```python
from build123d import *

# Parameters (mm, degrees)
BOSS_EXTRUDE1_DEPTH                           = 63.5
F_18_0_18_DIAMETER_HOLE1_D                    = 18
CBORE_FOR_4_SOCKET_HEAD_CAP_SCREW1_AT_2_COUNT = 2
CBORE_FOR_4_SOCKET_HEAD_CAP_SCREW1_AT_2_PITCH = 38.572873922
M5_CLEARANCE_HOLE1_D                          = 5.5
CBORE_FOR_5_16_HEX_MACHINE_SCREW1_D           = 8.4328
CBORE_FOR_5_16_HEX_MACHINE_SCREW1_CBORE_D     = 20.6375
CBORE_FOR_5_16_HEX_MACHINE_SCREW1_CBORE_DEPTH = 5.842
F_10_CLEARANCE_HOLE1_D                        = 5.1054
CUT_EXTRUDE1_DEPTH                            = 27.19375
CUT_EXTRUDE1_DEPTH_BACK                       = 27.19375


with BuildPart() as part:
    # Sketch1 → Boss-Extrude1 (new body)
    with BuildSketch(Plane.XY):
        Polygon((-26.19375, 0), (26.19375, 0), (26.19375, 9.525), (26.19375, 85.725), (19.05, 85.725), (19.05, 9.525), (-19.05, 9.525), (-19.05, 85.725), (-26.19375, 85.725), (-26.19375, 9.525), align=None)
    extrude(amount=BOSS_EXTRUDE1_DEPTH)

    # 18.0 _18_ Diameter Hole1 (through all)
    with Locations(Plane(origin=(26.19375, 0, 0), x_dir=(0, 0, -1), z_dir=(1, 0, 0))):
        with Locations((-28.575, 42.8625)):
            Hole(F_18_0_18_DIAMETER_HOLE1_D / 2)

    # Sketch13 → CBORE for _4 Socket Head Cap Screw1 (revolve, cut)
    with BuildSketch(Plane(origin=(-26.19375, 61.9125, 12.7), x_dir=(0, 0, 1), z_dir=(0, 1, 0))):
        Polygon((0, 0), (0, 42.382574487), (1.63195, 41.402), (1.63195, 2.8448), (2.77876, 2.8448), (2.77876, 0), align=None)
    cbore_for_4_socket_head_cap_screw1 = revolve(axis=Axis((-32.54375, 61.9125, 12.7), (1, 0, 0)), mode=Mode.SUBTRACT)

    # CBORE for _4 Socket Head Cap Screw1 at 2: CBORE for _4 Socket Head Cap Screw1 ×2
    with Locations(*[Vector(0, -0.195090322, 0.98078528) * (i * CBORE_FOR_4_SOCKET_HEAD_CAP_SCREW1_AT_2_PITCH) for i in range(1, CBORE_FOR_4_SOCKET_HEAD_CAP_SCREW1_AT_2_COUNT)]):
        add(cbore_for_4_socket_head_cap_screw1, mode=Mode.SUBTRACT)

    # Mirror1: CBORE for _4 Socket Head Cap Screw1 across Right Plane
    add(cbore_for_4_socket_head_cap_screw1.mirror(Plane(origin=(0, 0, 0), x_dir=(0, 0, -1), z_dir=(1, 0, 0))), mode=Mode.SUBTRACT)

    # Mirror1 copy 1 sketch → Mirror1 copy 1 (revolve, cut)
    with BuildSketch(Plane(origin=(26.19375, 54.387305606, 50.531706965), x_dir=(0, 0, 1), z_dir=(0, 1, 0))):
        Polygon((0, 0), (0, -42.382574487), (1.63195, -41.402), (1.63195, -2.8448), (2.77876, -2.8448), (2.77876, 0), align=None)
    revolve(axis=Axis((32.54375, 54.387305606, 50.531706965), (1, 0, 0)), mode=Mode.SUBTRACT)

    # M5 Clearance Hole1 (through all)
    with Locations(Plane.ZY.offset(26.19375)):
        with Locations((28.575, 67.862500038), (28.575, 17.862499962)):
            m5_clearance_hole1 = Hole(M5_CLEARANCE_HOLE1_D / 2)

    # Mirror2: M5 Clearance Hole1 across plane
    add(m5_clearance_hole1.mirror(Plane(origin=(0, 0, 0), x_dir=(0, 0, 1), z_dir=(1, 0, 0))), mode=Mode.SUBTRACT)

    # CBORE for 5_16 Hex Machine Screw1 (through all)
    with Locations(Plane(origin=(0, 9.525, 0), x_dir=(1, 0, 0), z_dir=(0, 1, 0))):
        with Locations((0, -47.625), (0, -15.875)):
            CounterBoreHole(CBORE_FOR_5_16_HEX_MACHINE_SCREW1_D / 2, CBORE_FOR_5_16_HEX_MACHINE_SCREW1_CBORE_D / 2, CBORE_FOR_5_16_HEX_MACHINE_SCREW1_CBORE_DEPTH)

    # 10 Clearance Hole1 (through all)
    with Locations(Plane.ZY.offset(26.19375)):
        with Locations((57.15, 16.66875), (50.8, 16.66875)):
            Hole(F_10_CLEARANCE_HOLE1_D / 2)

    # Sketch33 → Cut-Extrude1 (cut, two sides)
    with BuildSketch(Plane(origin=(0, 0, 0), x_dir=(0, 0, -1), z_dir=(1, 0, 0))) as cut_extrude1_sk:
        with BuildLine():
            Line((-63.5, 85.725), (-63.5, 9.525))
            ThreePointArc((-63.5, 9.525), (-63.350798487, 13.109275044), (-62.904226292, 16.66875))
            Line((-62.904226292, 16.66875), (-56.403219724, 55.373508453))
            ThreePointArc((-56.403219724, 55.373508453), (-55.465840296, 57.719209927), (-53.640248783, 59.465122647))
            Line((-53.640248783, 59.465122647), (-31.668525817, 72.915788375))
            ThreePointArc((-31.668525817, 72.915788375), (-29.144183386, 73.760097453), (-26.504966009, 73.414129013))
            Line((-26.504966009, 73.414129013), (-10.619918046, 67.491076629))
            ThreePointArc((-10.619918046, 67.491076629), (-8.052135843, 65.633335513), (-6.80142126, 62.721219352))
            Line((-6.80142126, 62.721219352), (-0.487438724, 16.66875))
            ThreePointArc((-0.487438724, 16.66875), (-0.122001188, 13.105180183), (0, 9.525))
            Line((0, 9.525), (0, 85.725))
            Line((0, 85.725), (-63.5, 85.725))
        make_face()
    extrude(amount=CUT_EXTRUDE1_DEPTH, mode=Mode.SUBTRACT)
    extrude(cut_extrude1_sk.sketch, amount=-CUT_EXTRUDE1_DEPTH_BACK, mode=Mode.SUBTRACT)


solid = part.part
```
The model under review builds one solid part; all positions refer to its coordinate system, in mm. A direction names the side the tool comes from. Coordinates: 2 decimals unless noted, no trailing zeros. Write each loop counter-clockwise with the first axis right and the second up, starting at its lowest first coordinate (ties: lowest second). Pieces come first, ordered by that corner, then holes. Notation, with made-up numbers: (25, 89) - (81, 89) arc R15 ccw to (81, 118) - close; hole circle Ø10 at (39, 57.25). An arc over 180 degrees is marked (long way). Answer in a Markdown table with one row per item. Add a question column.
Q1. Consider section C-C on y = 39. Give the boundary of the cut face in (x, z).
Q2. Consider section D-D on z = 21.5. Give the boundary of the cut face in (x, y) (3 decimals).
Q3. To check wall thickness, follow line 1 along X through (y, z) = (20, 40); line 2 along Y through (x, z) = (21.5, 50.8). State the ranges of each line that lie inside material, in increasing order. Write a range as from..to.
Q4. Consider section B-B on z = 12.7. Give the number of separate pieces and of enclosed holes in the cut face, then the cut area to 3 significant figures.
Q5. Consider section A-A on x = 0. Give the boundary of the cut face in (y, z) (3 decimals).
Q6. Draft analysis for pull direction Z (two halves, no side actions). For faces 5 (the face through (-22.572, 73.756, 29.182)), 6 (the face through (-26.194, 29, 31)), 7 (the face through (0, 3.683, 52)), state which applies: +Z half, -Z half, draft (parallel to the pull), parting line (faces both ways), or undercut.
Q7. For faces 1 (the face through (-1.343, 6.645, 37.394)), 2 (the face through (-23.349, 56, 49)), 3 (the face through (24.791, 59.157, 12.338)), 4 (the face through (21.23, 55.38, 49.237)), list the 3-axis set-ups (+Z, -Z, +X, -X, +Y, -Y) from which the entire face can be reached by the end or side of a thin tool; tool diameter is ignored.
Q8. Clearance check with flat-ended pins moving along their axes: pin 1 (4 mm diameter, centred on y = 61.91, z = 12.7, fed in from -X); pin 2 (4 mm diameter, centred on x = 18, z = 20, fed in from +Y); pin 3 (5 mm diameter, centred on y = 54.39, z = 50.53, fed in from +X). State where each tip first meets the part, or that it passes through.
Answers below:
| question | item | result |
|---|---|---|
| 1 | outline | (-26.19, 3.55) - (-19.05, 3.55) - (-19.05, 20.45) - (-26.19, 20.45) - close; (-26.19, 36.7) - (-19.05, 36.7) - (-19.05, 59.15) - (-26.19, 59.15) - close; (19.05, 3.55) - (26.19, 3.55) - (26.19, 20.45) - (19.05, 20.45) - close; (19.05, 36.7) - (26.19, 36.7) - (26.19, 59.15) - (19.05, 59.15) - close |
| 2 | outline | (-26.194, 0) - (26.194, 0) - (26.194, 37.3) - (19.05, 37.3) - (19.05, 9.525) - (8.651, 9.525) - (8.651, 3.683) - (-8.651, 3.683) - (-8.651, 9.525) - (-19.05, 9.525) - (-19.05, 37.3) - (-26.194, 37.3) - close; (-26.194, 48.425) - (-19.05, 48.425) - (-19.05, 71.548) - (-26.194, 71.548) - close; (19.05, 48.425) - (26.194, 48.425) - (26.194, 71.548) - (19.05, 71.548) - close |
| 3 | line 1 | -26.19..-19.05, 19.05..26.19 |
| 3 | line 2 | 0..14.12, 19.22..52.78, 56..61.2 |
| 4 | separate pieces | 4 |
| 4 | enclosed holes | 0 |
| 4 | area | 1,140 mm² |
| 5 | outline | (0, 0) - (9.525, 0) - (9.525, 5.556) - (3.683, 5.556) - (3.683, 11.659) - (0, 11.659) - close; (0, 20.091) - (3.683, 20.091) - (3.683, 26.194) - (9.525, 26.194) - (9.525, 37.306) - (3.683, 37.306) - (3.683, 43.409) - (0, 43.409) - close; (0, 51.841) - (3.683, 51.841) - (3.683, 57.944) - (9.525, 57.944) - (9.525, 63.5) - (0, 63.5) - close |
| 6 | face 5 | parting line |
| 6 | face 6 | draft |
| 6 | face 7 | undercut |
| 7 | face 1 | +Y |
| 7 | face 2 | -X |
| 7 | face 3 | +X |
| 7 | face 4 | +X, -X |
| 8 | pin 1 | x = -23.35 |
| 8 | pin 2 | y = 71.62 |
| 8 | pin 3 | x = 23.35 |
